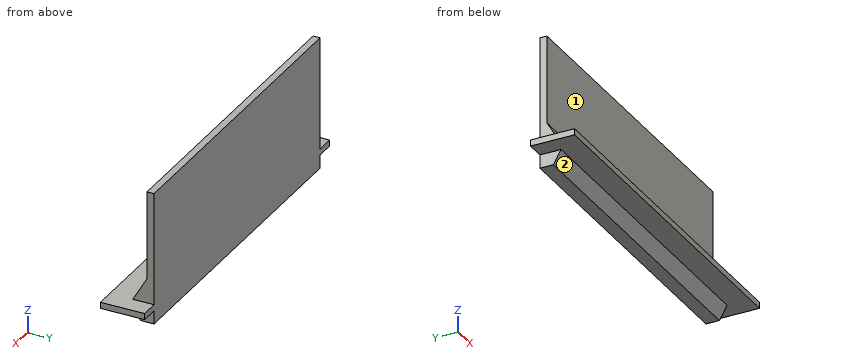
from build123d import *

# Parameters (mm, degrees)
SKETCH1_W           = 200.5
SKETCH1_H           = 3.5
BOSS_EXTRUDE1_DEPTH = 21
SKETCH3_W           = 180
SKETCH3_H           = 75
BOSS_EXTRUDE2_DEPTH = 4
CHAMFER1_SIZE       = 8
CHAMFER1_SIZE_2     = 13.856406461
SKETCH4_W           = 10.25
SKETCH4_H           = 3.5
BOSS_EXTRUDE3_DEPTH = 4


with BuildPart() as part:
    # Sketch1 → Boss-Extrude1 (new body)
    with BuildSketch(Plane(origin=(0, 0, 0), x_dir=(1, 0, 0), z_dir=(0, 1, 0))):
        Rectangle(SKETCH1_W, SKETCH1_H)
    extrude(amount=BOSS_EXTRUDE1_DEPTH)

    # Sketch3 → Boss-Extrude2 (add)
    with BuildSketch(Plane(origin=(0, 21, 0), x_dir=(1, 0, 0), z_dir=(0, 1, 0))):
        with Locations((0, -28.15)):
            Rectangle(SKETCH3_W, SKETCH3_H)
    extrude(amount=BOSS_EXTRUDE2_DEPTH)

    # Chamfer1
    # the kernel refuses this chamfer: 13.856406461, 8 mm, written as the material it adds along each edge
    with BuildSketch(Plane(origin=(-90, 21, -1.75), x_dir=(0, -0.9983227437537926, 0.0578938624026714), z_dir=(1, 0, 0))) as chamfer1_piece_1_section:
        Polygon((CHAMFER1_SIZE * 0.998322743754, CHAMFER1_SIZE * 0.0578938624027), (-CHAMFER1_SIZE_2 * 0.0578938624008, CHAMFER1_SIZE_2 * 0.998322743721), (0, 0), align=None)
    chamfer1_piece_1 = extrude(amount=180, mode=Mode.PRIVATE)
    chamfer1_piece_1 = split(chamfer1_piece_1, bisect_by=Plane(origin=(0, 17.958795912, -9.35), z_dir=(0, 0, 1)), keep=Keep.TOP, mode=Mode.PRIVATE)
    add(chamfer1_piece_1)
    with BuildSketch(Plane(origin=(90, 21, 1.75), x_dir=(0, -0.9983227437537926, -0.0578938624026714), z_dir=(-1, 0, 0))) as chamfer1_piece_2:
        Polygon((CHAMFER1_SIZE * 0.998322743754, CHAMFER1_SIZE * 0.0578938624027), (-CHAMFER1_SIZE_2 * 0.0578938624008, CHAMFER1_SIZE_2 * 0.998322743721), (0, 0), align=None)
    extrude(amount=180)

    # Sketch4 → Boss-Extrude3 (add)
    with BuildSketch(Plane(origin=(0, 21, 0), x_dir=(1, 0, 0), z_dir=(0, 1, 0))):
        with Locations((-95.125, 0)):
            Rectangle(SKETCH4_W, SKETCH4_H)
        with Locations((95.125, 0)):
            Rectangle(SKETCH4_W, SKETCH4_H)
    extrude(amount=BOSS_EXTRUDE3_DEPTH)


solid = part.part
Could you check a few things on this model? Use its own coordinates, in mm. Face numbers are marked on the shaded views. A direction names the side the tool comes from. Give positions to 0.01 mm unless a question says otherwise; leave off trailing zeros. Order: outer loops, then holes, each group sorted by start corner. A loop starts at its lowest first (then second) coordinate and runs counter-clockwise, first axis right, second up. Notation, with made-up numbers: (55, -1.5) - (114, -1.5) arc R35 cw to (114, 36.5) - close; hole circle Ø1 at (-31.5, -23.5). An arc over 180 degrees is marked (long way). Return JSON: item names as keys, results as strings. Group by question number.
Q1. Please list where these lines run through material, in increasing order: line 1 along Z through (x, y) = (42, 6); line 2 along Y through (x, z) = (26.5, 52); line 3 along X through (y, z) = (23.25, 54). Write a range as [from, to].
Q2. Will these pins go through, and if not, where does the flat tip stop? pin 1 Ø5 at (x, y) = (-19.5, 4.5) entering from -Z; pin 2 Ø1 at (x, y) = (-15, 17) entering from +Z; pin 3 Ø6 at (x, z) = (-38, 5.5) entering from -Y.
Q3. Suppose I cut it at C-C, the plane y = 2.75. Please give me the cut outline in (x, z).
Q4. Suppose I cut it at A-A, the plane x = -79.5. Please give me the cut outline in (y, z).
Q5. Which directions (+Z, -Z, +X, -X, +Y, -Y) give clear straight access to the entire face, cutting with the end or side of a thin tool? Please do the marked faces 1 and 2.
Q6. Suppose I cut it at B-B, the plane z = 19.5. Please give me the cut outline in (x, y), and give its area (3 significant figures).
Resolved:
{
 "1": {"line 1": "z = [-1.75, 1.75]", "line 2": "y = [21, 25]", "line 3": "x = [-90, 90]"},
 "2": {"pin 1": "stops at z = -1.75", "pin 2": "stops at z = 9.54", "pin 3": "stops at y = 13.43"},
 "3": {"outline": "(-100.25, -1.75) - (100.25, -1.75) - (100.25, 1.75) - (-100.25, 1.75) - close"},
 "4": {"outline": "(0, -1.75) - (13, -1.75) - (17.39, -9.35) - (25, -9.35) - (25, 65.65) - (21, 65.65) - (21, 15.61) - (13, 1.75) - (0, 1.75) - close"},
 "5": {"face 1": "+Z, +X, -X, -Y", "face 2": "-Z, +X, -X, -Y"},
 "6": {"outline": "(-90, 21) - (90, 21) - (90, 25) - (-90, 25) - close", "area": "720 mm2"}
}
